Verification items for the finished model (mm, model axes). Face numbers are marked on the shaded views. Give positions to 0.01 mm unless a question says otherwise; leave off trailing zeros. Write each loop counter-clockwise with the first axis right and the second up, starting at its lowest first coordinate (ties: lowest second). Pieces come first, ordered by that corner, then holes. Notation, with made-up numbers: M 68.25,-11 L 101.25,-11 A14 cw 101.25,0 Z; hole C 2.5,46.5 d1. An arc over 180 degrees is marked long. Answer as a JSON object with one key per item and string values.
```python
from build123d import *

# Parameters (mm, degrees)
SKETCH1_R           = 3
BOSS_EXTRUDE2_DEPTH = 6
CUT_EXTRUDE1_DEPTH  = 7
CUT_EXTRUDE2_DEPTH  = 7


with BuildPart() as part:
    # Sketch1 → Boss-Extrude2 (new body)
    with BuildSketch(Plane.XY):
        with BuildLine():
            Line((-129.483201213, -12.731798863), (-129.756040866, -10.003402327))
            ThreePointArc((-129.756040866, -10.003402327), (-131.945122685, -10.112584142), (-134.134204503, -10.003402327))
            Line((-134.134204503, -10.003402327), (-134.407044157, -12.731798863))
            ThreePointArc((-134.407044157, -12.731798863), (-142.137187462, -5.76575817), (-152.035027318, -2.554278039))
            Line((-152.035027318, -2.554278039), (-149.808586433, -0.9537937))
            ThreePointArc((-149.808586433, -0.9537937), (-150.997681568, 0.887415858), (-151.997668251, 2.837807232))
            Line((-151.997668251, 2.837807232), (-154.49694879, 1.709895035))
            ThreePointArc((-154.49694879, 1.709895035), (-152.329252239, 11.887415858), (-154.49694879, 22.064936682))
            Line((-154.49694879, 22.064936682), (-151.997668251, 20.937024485))
            ThreePointArc((-151.997668251, 20.937024485), (-150.997681568, 22.887415858), (-149.808586433, 24.728625416))
            Line((-149.808586433, 24.728625416), (-152.035027318, 26.329109756))
            ThreePointArc((-152.035027318, 26.329109756), (-142.137187462, 29.540589886), (-134.407044157, 36.506630579))
            Line((-134.407044157, 36.506630579), (-134.134204503, 33.778234043))
            ThreePointArc((-134.134204503, 33.778234043), (-131.945122685, 33.887415858), (-129.756040866, 33.778234043))
            Line((-129.756040866, 33.778234043), (-129.483201213, 36.506630579))
            ThreePointArc((-129.483201213, 36.506630579), (-121.753057907, 29.540589886), (-111.855218051, 26.329109756))
            Line((-111.855218051, 26.329109756), (-114.081658936, 24.728625416))
            ThreePointArc((-114.081658936, 24.728625416), (-112.892563801, 22.887415858), (-111.892577118, 20.937024485))
            Line((-111.892577118, 20.937024485), (-109.393296579, 22.064936682))
            ThreePointArc((-109.393296579, 22.064936682), (-111.56099313, 11.887415858), (-109.393296579, 1.709895035))
            Line((-109.393296579, 1.709895035), (-111.892577118, 2.837807232))
            ThreePointArc((-111.892577118, 2.837807232), (-112.892563801, 0.887415858), (-114.081658936, -0.9537937))
            Line((-114.081658936, -0.9537937), (-111.855218051, -2.554278039))
            ThreePointArc((-111.855218051, -2.554278039), (-121.753057907, -5.76575817), (-129.483201213, -12.731798863))
        make_face()
        with Locations((-131.945122685, 11.887415858)):
            Circle(SKETCH1_R, mode=Mode.SUBTRACT)
    extrude(amount=BOSS_EXTRUDE2_DEPTH)

    # Sketch2 → Cut-Extrude1 (cut, through all)
    with BuildSketch(Plane(origin=(0, 0, 0), x_dir=(-1, 0, 0), z_dir=(0, 0, -1))):
        with BuildLine():
            ThreePointArc((130.738332945, 29.846952186), (131.945122685, 29.887451596), (133.151912424, 29.846952186))
            Line((133.151912424, 29.846952186), (134.365507242, 32.447465558))
            Line((134.365507242, 32.447465558), (137.658457935, 32.842028481))
            ThreePointArc((137.658457935, 32.842028481), (135.942681801, 34.594415702), (134.407044157, 36.506630579))
            Line((134.407044157, 36.506630579), (134.134204503, 33.778234043))
            ThreePointArc((134.134204503, 33.778234043), (131.945122685, 33.887415858), (129.756040866, 33.778234043))
            Line((129.756040866, 33.778234043), (129.483201213, 36.506630579))
            ThreePointArc((129.483201213, 36.506630579), (127.947563568, 34.594415702), (126.231787434, 32.842028481))
            Line((126.231787434, 32.842028481), (129.524738127, 32.447465558))
            Line((129.524738127, 32.447465558), (130.738332945, 29.846952186))
        make_face()
        with BuildLine():
            Line((148.540455749, 24.263555222), (146.895142515, 21.912294593))
            ThreePointArc((146.895142515, 21.912294593), (147.533610903, 20.887433727), (148.101932254, 19.82207345))
            Line((148.101932254, 19.82207345), (150.960840307, 20.071326194))
            Line((150.960840307, 20.071326194), (152.949017168, 17.416828703))
            ThreePointArc((152.949017168, 17.416828703), (153.608740951, 19.778928032), (154.49694879, 22.064936682))
            Line((154.49694879, 22.064936682), (151.997668251, 20.937024485))
            ThreePointArc((151.997668251, 20.937024485), (150.997681568, 22.887415858), (149.808586433, 24.728625416))
            Line((149.808586433, 24.728625416), (152.035027318, 26.329109756))
            ThreePointArc((152.035027318, 26.329109756), (149.611181835, 26.702903528), (147.235681918, 27.312615637))
            Line((147.235681918, 27.312615637), (148.540455749, 24.263555222))
        make_face()
        with BuildLine():
            ThreePointArc((115.788313115, 19.82207345), (116.356634466, 20.887433727), (116.995102855, 21.912294593))
            Line((116.995102855, 21.912294593), (115.34978962, 24.263555222))
            Line((115.34978962, 24.263555222), (116.654563452, 27.312615637))
            ThreePointArc((116.654563452, 27.312615637), (114.279063535, 26.702903528), (111.855218051, 26.329109756))
            Line((111.855218051, 26.329109756), (114.081658936, 24.728625416))
            ThreePointArc((114.081658936, 24.728625416), (112.892563801, 22.887415858), (111.892577118, 20.937024485))
            Line((111.892577118, 20.937024485), (109.393296579, 22.064936682))
            ThreePointArc((109.393296579, 22.064936682), (110.281504418, 19.778928032), (110.941228201, 17.416828703))
            Line((110.941228201, 17.416828703), (112.929405062, 20.071326194))
            Line((112.929405062, 20.071326194), (115.788313115, 19.82207345))
        make_face()
        with BuildLine():
            Line((150.960840307, 3.703505522), (148.101932254, 3.952758266))
            ThreePointArc((148.101932254, 3.952758266), (147.533610903, 2.887397989), (146.895142515, 1.862537123))
            Line((146.895142515, 1.862537123), (148.540455749, -0.488723506))
            Line((148.540455749, -0.488723506), (147.235681918, -3.537783921))
            ThreePointArc((147.235681918, -3.537783921), (149.611181835, -2.928071812), (152.035027318, -2.554278039))
            Line((152.035027318, -2.554278039), (149.808586433, -0.9537937))
            ThreePointArc((149.808586433, -0.9537937), (150.997681568, 0.887415858), (151.997668251, 2.837807232))
            Line((151.997668251, 2.837807232), (154.49694879, 1.709895035))
            ThreePointArc((154.49694879, 1.709895035), (153.608740951, 3.995903684), (152.949017168, 6.358003014))
            Line((152.949017168, 6.358003014), (150.960840307, 3.703505522))
        make_face()
        with BuildLine():
            ThreePointArc((116.995102855, 1.862537123), (116.356634466, 2.887397989), (115.788313115, 3.952758266))
            Line((115.788313115, 3.952758266), (112.929405062, 3.703505522))
            Line((112.929405062, 3.703505522), (110.941228201, 6.358003014))
            ThreePointArc((110.941228201, 6.358003014), (110.281504418, 3.995903684), (109.393296579, 1.709895035))
            Line((109.393296579, 1.709895035), (111.892577118, 2.837807232))
            ThreePointArc((111.892577118, 2.837807232), (112.892563801, 0.887415858), (114.081658936, -0.9537937))
            Line((114.081658936, -0.9537937), (111.855218051, -2.554278039))
            ThreePointArc((111.855218051, -2.554278039), (114.279063535, -2.928071812), (116.654563452, -3.537783921))
            Line((116.654563452, -3.537783921), (115.34978962, -0.488723506))
            Line((115.34978962, -0.488723506), (116.995102855, 1.862537123))
        make_face()
        with BuildLine():
            Line((134.365507242, -8.672633842), (133.151912424, -6.072120469))
            ThreePointArc((133.151912424, -6.072120469), (131.945122685, -6.11261988), (130.738332945, -6.072120469))
            Line((130.738332945, -6.072120469), (129.524738127, -8.672633842))
            Line((129.524738127, -8.672633842), (126.231787434, -9.067196765))
            ThreePointArc((126.231787434, -9.067196765), (127.947563568, -10.819583986), (129.483201213, -12.731798863))
            Line((129.483201213, -12.731798863), (129.756040866, -10.003402327))
            ThreePointArc((129.756040866, -10.003402327), (131.945122685, -10.112584142), (134.134204503, -10.003402327))
            Line((134.134204503, -10.003402327), (134.407044157, -12.731798863))
            ThreePointArc((134.407044157, -12.731798863), (135.942681801, -10.819583986), (137.658457935, -9.067196765))
            Line((137.658457935, -9.067196765), (134.365507242, -8.672633842))
        make_face()
    extrude(amount=-CUT_EXTRUDE1_DEPTH, mode=Mode.SUBTRACT)

    # Sketch5 → Cut-Extrude2 (cut, through all)
    with BuildSketch(Plane(origin=(0, 0, 0), x_dir=(-1, 0, 0), z_dir=(0, 0, -1))):
        Polygon((130.20552592, 31.11947551), (129.574953313, 32.121497093), (129.310917186, 32.281735325), (128.697286189, 32.654135676), (127.366259017, 32.873895382), (126.416214667, 32.654135676), (126.147436582, 32.54260411), (125.218815368, 32.111317334), (126.147436582, 39.612839074), (129.890239616, 35.341275211), align=None)
        Polygon((137.742808787, 39.612839074), (134.000005753, 35.341275211), (133.68471945, 31.11947551), (134.315292057, 32.121497093), (134.579328183, 32.281735325), (135.19295918, 32.654135676), (136.523986352, 32.873895382), (137.474030702, 32.654135676), (137.742808787, 32.54260411), (138.671430002, 32.111317334), align=None)
        Polygon((151.553547848, 19.458066854), (152.409378922, 18.415243363), (152.694083609, 17.482600968), (152.731883481, 17.194066536), (152.822688785, 16.174213586), (158.854886572, 20.729184019), (153.284202235, 21.834764595), (149.470373293, 19.996910693), (150.653435743, 19.951829588), (150.924224185, 19.803286711), align=None)
        Polygon((148.290018687, 24.365864472), (148.305711352, 25.083484679), (147.830515254, 26.346067876), (147.165175591, 27.058950565), (146.934197379, 27.235953431), (146.096381468, 27.824519606), (153.05720047, 30.771070914), (151.229319167, 25.393926474), (147.730776528, 23.009980675), (148.283266371, 24.057083363), align=None)
        Polygon((148.305711352, -1.308652963), (147.830515254, -2.57123616), (147.165175591, -3.284118849), (146.934197379, -3.461121715), (146.096381468, -4.04968789), (153.05720047, -6.996239198), (151.229319167, -1.619094757), (147.730776528, 0.764851041), (148.283266371, -0.282251647), (148.290018687, -0.591032756), align=None)
        Polygon((150.924224185, 3.971545005), (151.553547848, 4.316764862), (152.409378922, 5.359588353), (152.694083609, 6.292230748), (152.731883481, 6.58076518), (152.822688785, 7.60061813), (158.854886572, 3.045647698), (153.284202235, 1.940067121), (149.470373293, 3.777921023), (150.653435743, 3.823002128), align=None)
        Polygon((128.697286189, -8.87930396), (127.366259017, -9.099063665), (126.416214667, -8.87930396), (126.147436582, -8.767772393), (125.218815368, -8.336485618), (126.147436582, -15.838007358), (129.890239616, -11.566443495), (130.20552592, -7.344643794), (129.574953313, -8.346665377), (129.310917186, -8.506903609), align=None)
        Polygon((134.579328183, -8.506903609), (135.19295918, -8.87930396), (136.523986352, -9.099063665), (137.474030702, -8.87930396), (137.742808787, -8.767772393), (138.671430002, -8.336485618), (137.742808787, -15.838007358), (134.000005753, -11.566443495), (133.68471945, -7.344643794), (134.315292057, -8.346665377), align=None)
        Polygon((112.336697522, 4.316764862), (111.480866448, 5.359588353), (111.19616176, 6.292230748), (111.158361888, 6.58076518), (111.067556584, 7.60061813), (105.035358798, 3.045647698), (110.606043134, 1.940067121), (114.419872076, 3.777921023), (113.236809627, 3.823002128), (112.966021184, 3.971545005), align=None)
        Polygon((115.600226683, -0.591032756), (115.584534017, -1.308652963), (116.059730115, -2.57123616), (116.725069778, -3.284118849), (116.95604799, -3.461121715), (117.793863901, -4.04968789), (110.8330449, -6.996239198), (112.660926203, -1.619094757), (116.159468841, 0.764851041), (115.606978999, -0.282251647), align=None)
        Polygon((115.584534017, 25.083484679), (116.059730115, 26.346067876), (116.725069778, 27.058950565), (116.95604799, 27.235953431), (117.793863901, 27.824519606), (110.8330449, 30.771070914), (112.660926203, 25.393926474), (116.159468841, 23.009980675), (115.606978999, 24.057083363), (115.600226683, 24.365864472), align=None)
        Polygon((112.966021184, 19.803286711), (112.336697522, 19.458066854), (111.480866448, 18.415243363), (111.19616176, 17.482600968), (111.158361888, 17.194066536), (111.067556584, 16.174213586), (105.035358798, 20.729184019), (110.606043134, 21.834764595), (114.419872076, 19.996910693), (113.236809627, 19.951829588), align=None)
    extrude(amount=-CUT_EXTRUDE2_DEPTH, mode=Mode.SUBTRACT)


solid = part.part
```
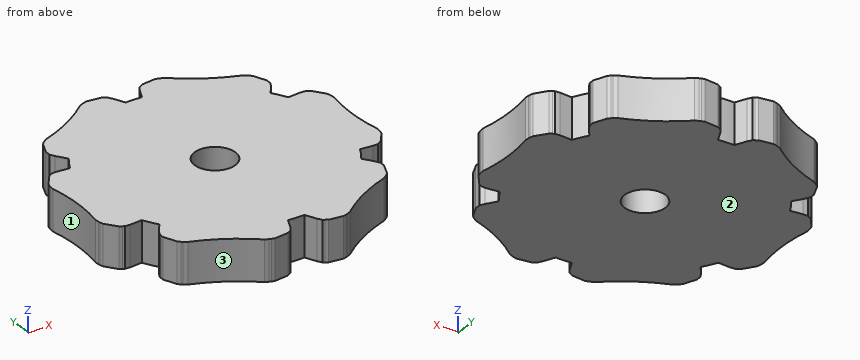
1) Section check C-C on y = 28.5. Record the boundary of the cut face in (x, z).
Completed:
{"outline": "M -144.14,0 L -119.75,0 L -119.75,6 L -144.14,6 Z"}
2) Release check for a two-part mould opening along Y. For the marked faces 1, 2 and 3 record: pulls with the +Y half, pulls with the -Y half, needs draft (parallel to the pull), parting line crosses it, or undercut.
Completed:
{"face 1": "undercut", "face 2": "needs draft", "face 3": "pulls with the -Y half"}
3) Section check A-A on y = 14. Record the boundary of the cut face in (x, z).
Completed:
{"outline": "M -152.42,0 L -134.08,0 L -134.08,6 L -152.42,6 Z; M -129.82,0 L -111.47,0 L -111.47,6 L -129.82,6 Z"}
4) Thickness scan on L1, parallel to Y at x = -116, z = 5.25; L2, parallel to Y at x = -148, z = 5; L3, parallel to Y at x = -113, z = 1.75. Record the ranges inside material, lowest first.
Completed:
{"L1": "y = -2.01 to 0.44, 3.54 to 20.24, 23.33 to 25.78", "L2": "y = -1.75 to 0.25, 3.75 to 20.03, 23.52 to 25.53", "L3": "y = 3.95 to 19.82"}
5) Section check B-B on x = -140.5. Record the boundary of the cut face in (y, z), and give its area (3 significant figures).
Completed:
{"outline": "M -6.8,0 L 30.57,0 L 30.57,6 L -6.8,6 Z", "area": "224 mm2"}
